Check sheet for the modelled part. Datum: model origin and axes. Units: mm. A direction names the side the tool comes from. Give positions to 0.01 mm unless a question says otherwise; leave off trailing zeros. Write each loop counter-clockwise with the first axis right and the second up, starting at its lowest first coordinate (ties: lowest second). Pieces come first, ordered by that corner, then holes. Notation, with made-up numbers: M 51.5,28.25 L 109.5,28.25 A5 ccw 109.5,32.25 Z; hole C 89,25 d11. An arc over 180 degrees is marked long. One line per item, written item: value. Start each with the question number.
from build123d import *

# Parameters (mm, degrees)
CUT_EXTRUDE1_DEPTH  = 50
CUT_EXTRUDE2_DEPTH  = 50
BOSS_EXTRUDE1_DEPTH = 5
BOSS_EXTRUDE2_DEPTH = 5


with BuildPart() as part:
    # Sketch4 → Revolve-Thin1 (revolve)
    with BuildSketch(Plane.XY):
        with BuildLine():
            ThreePointArc((0, 48.490566038), (50, -1.509433962), (0, -51.509433962))
            Line((0, -51.509433962), (0, -41.509433962))
            ThreePointArc((0, -41.509433962), (40, -1.509433962), (0, 38.490566038))
            Line((0, 38.490566038), (0, 48.490566038))
        make_face()
    revolve(axis=Axis((0, 48.490566038, 0), (0, -1, 0)))

    # Sketch5 → Cut-Extrude1 (cut)
    with BuildSketch(Plane.XY):
        Polygon((-30.644001245, -9.970067303), (-40.033240684, -26.272263251), (-40.033240684, 6.332128646), (-36.976129891, 0), (-30.644001245, 6.332128646), (-22.492903271, -1.818969328), (-14.341805297, 6.332128646), (-6.190707322, -1.818969328), (1.960390652, 6.332128646), (10.111488626, -1.818969328), (18.262586601, 6.332128646), (26.413684575, -1.818969328), (34.56478255, 6.332128646), (34.56478255, -9.970067303), (34.56478255, -26.272263251), (26.413684575, -18.121165277), (18.262586601, -9.970067303), (10.111488626, -18.121165277), (1.960390652, -9.970067303), (-6.190707322, -18.121165277), (-14.341805297, -9.970067303), (-22.492903271, -18.121165277), align=None)
    extrude(amount=CUT_EXTRUDE1_DEPTH, mode=Mode.SUBTRACT)

    # Sketch6 → Cut-Extrude2 (cut)
    with BuildSketch(Plane.XY):
        with BuildLine():
            add(Edge.make_bspline(
                [(-31.159893522, 26.245570533), (-30.561812418, 20.967271985), (-10.609739532, 12.440512153), (-22.402808053, 39.879513697), (-31.550689585, 29.694497906), (-31.159893522, 26.245570533)],
                knots=[0, 0, 0, 0, 0.370756889, 0.75774133, 1, 1, 1, 1], degree=3))
        make_face()
        with BuildLine():
            add(Edge.make_bspline(
                [(23.937401646, 19.642149389), (26.561792049, 18.17132991), (37.050887315, 25.488164902), (23.054790304, 40.061439696), (20.519151547, 21.557881447), (23.937401646, 19.642149389)],
                knots=[0, 0, 0, 0, 0.312357954, 0.593155955, 1, 1, 1, 1], degree=3))
        make_face()
    extrude(amount=CUT_EXTRUDE2_DEPTH, mode=Mode.SUBTRACT)

    # Sketch8 → Boss-Extrude1 (add)
    with BuildSketch(Plane.XY):
        with BuildLine():
            Line((-21.178417491, 37.628203487), (-11.569674779, 45.482179937))
            add(Edge.make_bspline(
                [(-11.569674779, 45.482179937), (-40.321950535, 80.658402053), (-45.12632189, 76.731413828), (-49.930693246, 72.804425603), (-21.178417491, 37.628203487)],
                knots=[4.71238898, 4.71238898, 4.71238898, 6.283185307, 6.283185307, 7.853981634, 7.853981634, 7.853981634], degree=2, weights=[1, 0.707106781, 1, 0.707106781, 1]))
        make_face()
    extrude(amount=BOSS_EXTRUDE1_DEPTH)

    # Sketch9 → Boss-Extrude2 (add)
    with BuildSketch(Plane.XY):
        with BuildLine():
            Line((14.416361682, 48.876227224), (6.987253857, 40.013654036))
            Line((6.987253857, 40.013654036), (17.559883218, 31.151080848))
            Line((17.559883218, 31.151080848), (24.988991043, 40.013654036))
            add(Edge.make_bspline(
                [(24.988991043, 40.013654036), (52.645598361, 73.0066745), (47.35928368, 77.437961094), (42.072969, 81.869247688), (14.416361682, 48.876227224)],
                knots=[4.71238898, 4.71238898, 4.71238898, 6.283185307, 6.283185307, 7.853981634, 7.853981634, 7.853981634], degree=2, weights=[1, 0.707106781, 1, 0.707106781, 1]))
        make_face()
    extrude(amount=BOSS_EXTRUDE2_DEPTH)


solid = part.part
1) Cross-section at C-C (x = 29.5). State how many separate pieces and enclosed holes the cut face has, plus the area to 3 significant figures.
2) Gauge pin test, flat ends, axial feed: pin 1 (10 mm diameter, centred on y = -4.5, z = 23.5, fed in from -X); pin 2 (7.5 mm diameter, centred on x = -26.5, y = 29, fed in from +Z); pin 3 (4 mm diameter, centred on x = 33, z = -24.5, fed in from +Y). Record the tip position at first contact, or that the pin passes through.
3) Material ranges on L1, parallel to Y at x = -21.5, z = -13; L2, parallel to X at y = -12.5, z = -26; L3, parallel to Y at x = 5, z = -31, recorded low to high. Write a range as from..to.
4) Cross-section at D-D (x = 4). Record the boundary of the cut face in (y, z).
5) Tool access check on faces 3 (the flat face through (16, 34, 0)), 4 (the flat face through (-30, 57, 5)), 5 (the flat face through (-30, 57, 0)), 6 (the flat face through (14.13, 2.2, 41.74)). Record the directions out of +Z, -Z, +X, -X, +Y, -Y that give a thin tool (end or side, any length) a straight path to the whole face; none if there is none.
6) Cross-section at B-B (z = -16). Record the boundary of the cut face in (x, y), plus the area to 3 significant figures.
7) Cross-section at A-A (y = -36). Record the boundary of the cut face in (x, z), plus the area to 3 significant figures.
8) Draft check along X on faces 1 (the flat face through (31, 59, 0)), 2 (the flat face through (30.43, 2.2, 32.99)). Enter one of: released by +X, released by -X, zero draft, split by the parting line, or undercut.
Data:
1. separate pieces: 3
1. enclosed holes: 0
1. area: 2,330 mm2
2. pin 1: stops at x = -46.38
2. pin 2: stops at z = 24.19
2. pin 3: stops at y = 29.65
3. L1: y = -44.74..-32.63, 29.62..41.72
3. L2: x = -41.27..-28.34, 28.34..41.27
3. L3: y = -40.42..-26.29, 23.27..37.4
4. outline: M -12.01,38.39 L -12.01,48.72 A49.84 ccw long 4.29,49.5 L 4.29,39.37 A39.8 cw long Z
5. face 3: none
5. face 4: +Z, -X, +Y
5. face 5: -Z, -X, +Y
5. face 6: +Z
6. outline: C 0,-1.51 d94.74; hole C 0,-1.51 d73.32
6. area: 2,830 mm2
7. outline: C 0,0 d72.4; hole C 0,0 d40.52
7. area: 2,830 mm2
8. face 1: zero draft
8. face 2: undercut
